For this review, use the dimensioned drawing (mm, ordinates from the lowest corner) and the shaded views. A direction names the side the tool comes from. Round coordinates to 2 decimals unless told otherwise and drop trailing zeros. Loops run counter-clockwise (first coordinate to the right, second up) from the corner with the lowest first, then second, coordinate; pieces in that order, holes last. Notation, with made-up numbers: M 70.25,28.5 L 105.25,28.5 A10 cw 105.25,43.5 Z; hole C 47.25,5.5 d1. An arc over 180 degrees is marked long. Answer as a JSON object with one key per item and string values. Group by question number.
Item 1: Insertion check: P1, Ø4, axis at x = 33.5, y = 13.5, coming from the -Z side; P2, Ø3, axis at x = 39, y = 7, coming from the -Z side; P3, Ø17.5, axis at x = 36.53, y = 40.38, coming from the +Z side; P4, Ø6.5, axis at y = 3.5, z = 21, coming from the +X side. Each pin has a flat end and moves straight along its axis. Give the tip position at first contact, or say it passes through.
Item 2: Consider section A-A (y = 43.5). Give the boundary of the cut face in (x, z) (1 decimal).
Item 3: Tool access review of the marked faces 4, 5, 6, 7 and 8: name each direction out of +Z, -Z, +X, -X, +Y, -Y from which nothing blocks a thin tool from reaching the whole face with its end or side.
Item 4: Consider section C-C (z = 18). Give the boundary of the cut face in (x, y) (1 decimal).
Item 5: Consider section D-D (x = 49). Give the boundary of the cut face in (y, z).
Item 6: The part is to be moulded in two halves that separate along Y. For the marked faces 1, 2 and 3, say which applies: +Y half, -Y half, draft (parallel to the pull), parting line (faces both ways), or undercut.
Item 7: Consider section B-B (x = 33.5). Give the boundary of the cut face in (y, z).
Item 8: To check wall thickness, follow line 1 (X direction, y = 20, z = 37.5); line 2 (Y direction, x = 31, z = 47.5) (1 decimal). State the ranges of each line that lie inside material, in increasing order.
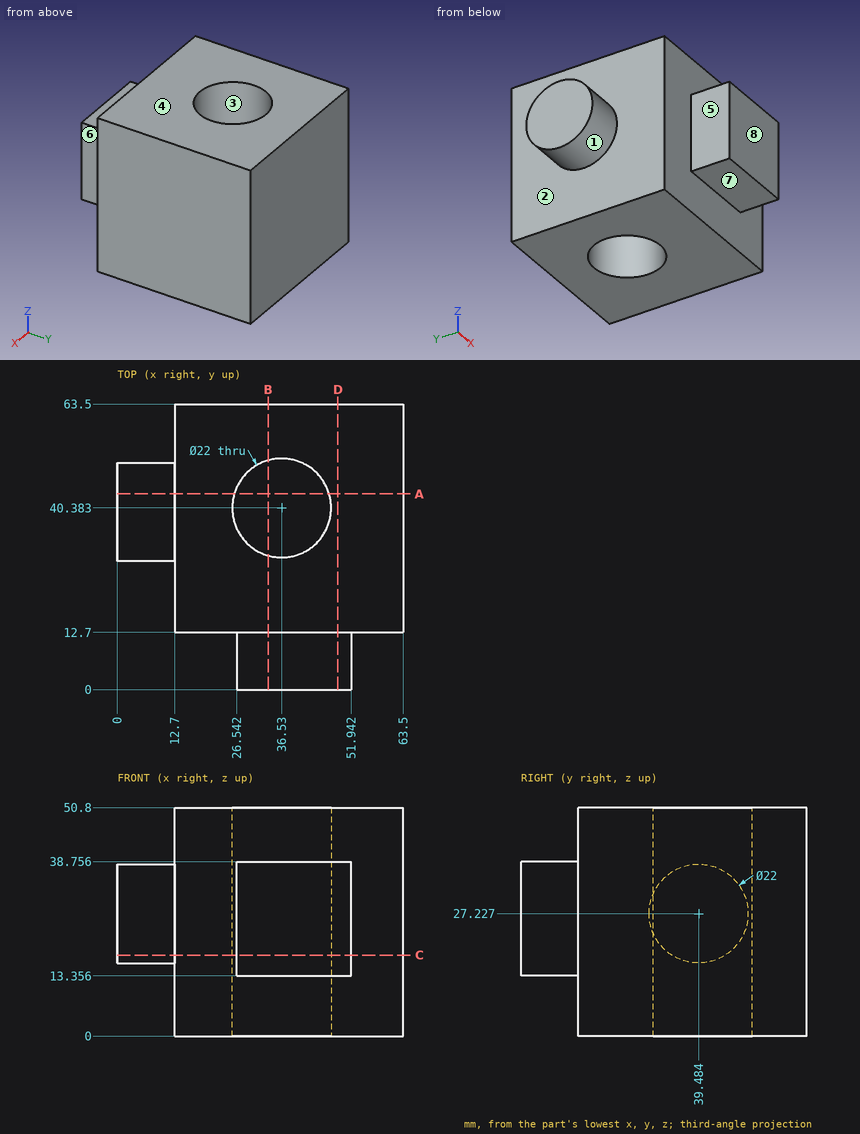
Geometry results:
{
 "1": {"P1": "stops at z = 0", "P2": "stops at z = 13.36", "P3": "passes through", "P4": "stops at x = 51.94"},
 "2": {"outline": "M 0,17 L 12.7,17 L 12.7,0 L 26,0 L 26,50.8 L 12.7,50.8 L 12.7,37.5 L 0,37.5 Z; M 47.1,0 L 63.5,0 L 63.5,50.8 L 47.1,50.8 Z"},
 "3": {"face 4": "+Z, +X, -X, +Y, -Y", "face 5": "+Z, -Z, -X, -Y", "face 6": "+Z, -Z, +X, -Y", "face 7": "-Z, +X, -X, -Y", "face 8": "+Z, -Z, +X, -X, -Y"},
 "4": {"outline": "M 0,33.5 L 12.7,33.5 L 12.7,12.7 L 26.5,12.7 L 26.5,0 L 51.9,0 L 51.9,12.7 L 63.5,12.7 L 63.5,63.5 L 12.7,63.5 L 12.7,45.5 L 0,45.5 Z; hole C 36.5,40.4 d22"},
 "5": {"outline": "M 0,13.36 L 12.7,13.36 L 12.7,0 L 63.5,0 L 63.5,50.8 L 12.7,50.8 L 12.7,38.76 L 0,38.76 Z"},
 "6": {"face 1": "parting line", "face 2": "draft", "face 3": "undercut"},
 "7": {"outline": "M 0,13.36 L 12.7,13.36 L 12.7,0 L 29.81,0 L 29.81,50.8 L 12.7,50.8 L 12.7,38.76 L 0,38.76 Z; M 50.96,0 L 63.5,0 L 63.5,50.8 L 50.96,50.8 Z"},
 "8": {"line 1": "x = 12.7 to 63.5", "line 2": "y = 12.7 to 30.9, 49.9 to 63.5"}
}
